CAD build for the part. Positions are in the model's coordinates, mm. Give positions to 0.01 mm unless a question says otherwise; leave off trailing zeros. Order: outer loops, then holes, each group sorted by start corner. A loop starts at its lowest first (then second) coordinate and runs counter-clockwise, first axis right, second up. Notation, with made-up numbers: (-32.5, -6) -> (20.5, -6) arc R16 cw to (20.5, 12) -> close; hole circle Ø8 at (63.25, -32.75). An arc over 180 degrees is marked (long way). Answer as CSV lines item,"result".
```python
from build123d import *

# Parameters (mm, degrees)
SKETCH1_W           = 93
SKETCH1_H           = 50
BOSS_EXTRUDE1_DEPTH = 2
SKETCH2_R           = 1.25
CUT_EXTRUDE1_DEPTH  = 2
SKETCH3_R           = 1.6
CUT_EXTRUDE2_DEPTH  = 2


with BuildPart() as part:
    # Sketch1 → Boss-Extrude1 (new body)
    with BuildSketch(Plane(origin=(0, 0, 0), x_dir=(1, 0, 0), z_dir=(0, 1, 0))):
        Rectangle(SKETCH1_W, SKETCH1_H)
    extrude(amount=BOSS_EXTRUDE1_DEPTH)

    # Sketch2 → Cut-Extrude1 (cut)
    with BuildSketch(Plane(origin=(0, 2, 0), x_dir=(1, 0, 0), z_dir=(0, 1, 0))):
        with Locations((-44, 22.5)):
            Circle(SKETCH2_R)
        with Locations((44, 22.5)):
            Circle(SKETCH2_R)
        with Locations((44, -22.5)):
            Circle(SKETCH2_R)
        with Locations((-44, -22.5)):
            Circle(SKETCH2_R)
    extrude(amount=-CUT_EXTRUDE1_DEPTH, mode=Mode.SUBTRACT)

    # Sketch3 → Cut-Extrude2 (cut)
    with BuildSketch(Plane(origin=(0, 2, 0), x_dir=(1, 0, 0), z_dir=(0, 1, 0))):
        with Locations((-38.5, 16.5)):
            Circle(SKETCH3_R)
        with Locations((-38.5, -16.5)):
            Circle(SKETCH3_R)
        with Locations((38.5, 16.5)):
            Circle(SKETCH3_R)
        with Locations((38.5, -16.5)):
            Circle(SKETCH3_R)
    extrude(amount=-CUT_EXTRUDE2_DEPTH, mode=Mode.SUBTRACT)


solid = part.part
```
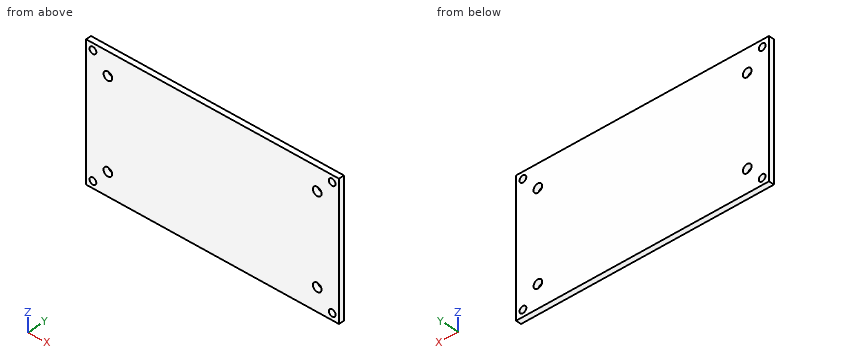
1) Wall check: line 1 along Z through (x, y) = (-38.5, 0.7); line 2 along X through (y, z) = (1.5, 22.5); line 3 along X through (y, z) = (1.1, -16.5). Give the ranges that are in metal, low to high. Write a range as [from, to].
Data:
line 1,"z = [-25, -18.1], [-14.9, 14.9], [18.1, 25]"
line 2,"x = [-46.5, -45.25], [-42.75, 42.75], [45.25, 46.5]"
line 3,"x = [-46.5, -40.1], [-36.9, 36.9], [40.1, 46.5]"
2) Band-saw the part on A-A, the plane x = -44. Write the cut outline in (y, z).
Data:
outline,"(0, -25) -> (2, -25) -> (2, -23.75) -> (0, -23.75) -> close; (0, -21.25) -> (2, -21.25) -> (2, 21.25) -> (0, 21.25) -> close; (0, 23.75) -> (2, 23.75) -> (2, 25) -> (0, 25) -> close"
3) Band-saw the part on B-B, the plane z = -22.5. Write the cut outline in (x, y), then the cut area to 3 significant figures.
Data:
outline,"(-46.5, 0) -> (-45.25, 0) -> (-45.25, 2) -> (-46.5, 2) -> close; (-42.75, 0) -> (42.75, 0) -> (42.75, 2) -> (-42.75, 2) -> close; (45.25, 0) -> (46.5, 0) -> (46.5, 2) -> (45.25, 2) -> close"
area,"176 mm2"
4) Pin check, flat tip, straight feed: P1, Ø1.5, axis at x = -26, z = 4, coming from the -Y side. Stop position of the tip, or through.
Data:
P1,"stops at y = 0"
